Source: CAD feature listing. Evaluate the final solid. Frame: model axes, mm. A direction names the side the tool comes from. Give positions to 0.01 mm unless a question says otherwise; leave off trailing zeros. Write each loop counter-clockwise with the first axis right and the second up, starting at its lowest first coordinate (ties: lowest second). Pieces come first, ordered by that corner, then holes. Notation, with made-up numbers: M -24.75,-29 L -6.75,-29 A28 cw -6.75,-4 Z; hole C -27.75,-7 d9. An arc over 180 degrees is marked long. Answer as a JSON object with one key per item and string values. Group by question number.
```python
from build123d import *

# Parameters (mm, degrees)
F1_DEPTH  = 41
F2_R      = 24.5503927786
F2_R_2    = 16.3
F3_DEPTH  = 25
F4_R      = 24.0523887052
F4_R_2    = 15
F5_DEPTH  = 9
F6_R      = 16.3
F7_DEPTH  = 7
F8_R      = 2.85
F9_DEPTH  = 41.001
F10_R     = 13.8
F11_DEPTH = 2.3
F12_R     = 6
F13_DEPTH = 41.001
F14_R     = 6.5
F15_DEPTH = 29
F16_R     = 2.5
F17_DEPTH = 13
F18_R     = 2.5
F19_DEPTH = 13
F21_D     = 4.2
F21_DEPTH = 8
F21_TIP   = 1.2618073
F22_R     = 3
F23_DEPTH = 29


with BuildPart() as f1:
    # F0 (on Front) → F1 (new body)
    with BuildSketch(Plane.XZ):
        Polygon((0, -20.7846096908), (18, -10.3923048454), (18, 10.3923048454), (0, 20.7846096908), (-18, 10.3923048454), (-18, -10.3923048454), align=None)
    extrude(amount=-F1_DEPTH)

    # F2 (on face) → F3 (cut)
    with BuildSketch(Plane(origin=(0, 41, 0), x_dir=(-1, 0, 0), z_dir=(0, 1, 0))):
        Circle(F2_R)
        Circle(F2_R_2, mode=Mode.SUBTRACT)
    extrude(amount=-F3_DEPTH, mode=Mode.SUBTRACT)

    # F4 (on face) → F5 (cut)
    with BuildSketch(Plane(origin=(0, 41, 0), x_dir=(-1, 0, 0), z_dir=(0, 1, 0))):
        Circle(F4_R)
        Circle(F4_R_2, mode=Mode.SUBTRACT)
    extrude(amount=-F5_DEPTH, mode=Mode.SUBTRACT)

    # F6 (on face) → F7 (join)
    with BuildSketch(Plane(origin=(0, 41, 0), x_dir=(-1, 0, 0), z_dir=(0, 1, 0))):
        Circle(F6_R)
    extrude(amount=-F7_DEPTH)

    # F8 (on face) → F9 (cut, through all)
    with BuildSketch(Plane.XZ):
        with Locations((4.87, -6.95)):
            Circle(F8_R)
        with Locations((8.5, 0)):
            Circle(F8_R)
    extrude(amount=-F9_DEPTH, mode=Mode.SUBTRACT)

    # F10 (on face) → F11 (cut)
    with BuildSketch(Plane(origin=(0, 41, 0), x_dir=(-1, 0, 0), z_dir=(0, 1, 0))):
        Circle(F10_R)
    extrude(amount=-F11_DEPTH, mode=Mode.SUBTRACT)

    # F12 (on face) → F13 (cut, through all)
    with BuildSketch(Plane.XZ):
        with Locations((-5, 0)):
            Circle(F12_R)
    extrude(amount=-F13_DEPTH, mode=Mode.SUBTRACT)

    # F14 (on face) → F15 (cut)
    with BuildSketch(Plane(origin=(0, 38.7, 0), x_dir=(-1, 0, 0), z_dir=(0, 1, 0))):
        with Locations((5, 0)):
            Circle(F14_R)
    extrude(amount=-F15_DEPTH, mode=Mode.SUBTRACT)

    # F16 (on face) → F17 (cut)
    with BuildSketch(Plane.XZ):
        with Locations((0, 14.7801668913)):
            Circle(F16_R)
    extrude(amount=-F17_DEPTH, mode=Mode.SUBTRACT)

    # F18 (on face) → F19 (cut)
    with BuildSketch(Plane.XZ):
        with Locations((0, -14.7801668913)):
            Circle(F18_R)
    extrude(amount=-F19_DEPTH, mode=Mode.SUBTRACT)

    # F21
    with Locations(Plane(origin=(9, 0, 15.5884572681), x_dir=(0.8660254038, 0, -0.5), z_dir=(0.5, 0, 0.8660254038))):
        with Locations((4.4923048454, 5.9)):
            Hole(F21_D / 2, depth=F21_DEPTH)
            with Locations((0, 0, -(F21_DEPTH + F21_TIP / 2))):  # 118° drill point
                Cone(0, F21_D / 2, F21_TIP, mode=Mode.SUBTRACT)

    # F22 (on face) → F23 (cut)
    with BuildSketch(Plane(origin=(0, 38.7, 0), x_dir=(-1, 0, 0), z_dir=(0, 1, 0))):
        with Locations((-4.62, 7.15)):
            Circle(F22_R)
    extrude(amount=-F23_DEPTH, mode=Mode.SUBTRACT)


solid = f1.part
```
(1) Section A-A, the plane x = 4.87. Return loops of the section in (y, z), plus the area to 3 significant figures.
(2) Section C-C, the plane y = 38. Return loops of the section in (x, z), plus the area to 3 significant figures.
(3) Contact query for flat-ended pins moving along their axis: pin 1 Ø1.5 at (x, y) = (6, 23) entering from -Z; pin 2 Ø1.5 at (x, y) = (5.5, 33.5) entering from -Z; pin 3 Ø3 at (x, z) = (4, 6.5) entering from +Y. Output: stop coordinate, or through.
(4) Ray query, L1, parallel to Z at x = 4, y = 25; L2, parallel to Y at x = 12.5, z = -13.5; L3, parallel to Y at x = -11, z = 11. Return the intervals inside material, ascending. Write a range as [from, to].
(5) Section B-B, the plane z = 0. State how many separate pieces and enclosed holes the cut face has, plus the area to 3 significant figures.
(6) Access query for faces 4 (the cylindrical face through (7.503, 19.079, -8.042)), 5 (the flat face through (-4.8, 32, -14.4)), 6 (the cylindrical face through (12.935, 24.112, -9.918)), 7 (the cylindrical face through (-0.54, 6.41, 12.34)). Directions: +Z, -Z, +X, -X, +Y, -Y. A direction counts if a zero-diameter tool reaches every point of the face in a straight line with its end or side. Return the directions, or none.
(7) Section D-D, the plane z = 18. Return loops of the section in (x, y), plus the area to 3 significant figures.
(8) Pull-direction query (X, two-part tool) for faces 1 (the flat face through (5, 9.7, 7)), 2 (the flat face through (9.126, 7.888, 15.516)), 3 (the flat face through (-18, 8, 0)); classes: pulls with the +X half, pulls with the -X half, needs draft (parallel to the pull), parting line crosses it, or undercut.
Reported:
{
 "1": {"outline": "M 0,-17.97 L 16,-17.97 L 16,-15.56 L 32,-15.56 L 32,-14.19 L 34,-14.19 L 34,-15.56 L 41,-15.56 L 41,-12.91 L 38.7,-12.91 L 38.7,-9.8 L 0,-9.8 Z; M 0,-4.1 L 38.7,-4.1 L 38.7,4.16 L 9.7,4.16 L 9.7,10.14 L 38.7,10.14 L 38.7,12.91 L 41,12.91 L 41,15.56 L 34,15.56 L 34,14.19 L 32,14.19 L 32,15.56 L 16,15.56 L 16,17.97 L 0,17.97 Z", "area": "894 mm2"},
 "2": {"outline": "C 0,0 d32.6; hole C -5,0 d13; hole C 4.62,7.15 d6; hole C 4.87,-6.95 d5.7; hole C 8.5,0 d5.7", "area": "623 mm2"},
 "3": {"pin 1": "stops at z = -15.43", "pin 2": "stops at z = -15.53", "pin 3": "stops at y = 9.7"},
 "4": {"L1": "z = [-15.8, -9.66], [-4.24, 4.21], [10.09, 15.8]", "L2": "y = [0, 16]", "L3": "y = [0, 32], [34, 41]"},
 "5": {"separate pieces": "3", "enclosed holes": "0", "area": "608 mm2"},
 "6": {"face 4": "+Y, -Y", "face 5": "none", "face 6": "+Y", "face 7": "-Y"},
 "7": {"outline": "M -4.82,0 L 4.82,0 L 4.82,16 L -4.82,16 Z", "area": "154 mm2"},
 "8": {"face 1": "undercut", "face 2": "pulls with the +X half", "face 3": "pulls with the -X half"}
}
